```python
from build123d import *

# Parameters (mm, degrees)
SKETCH_1_W          = 200
SKETCH_1_H          = 240
SKETCH_1_R          = 3.25
EXTRUDE_1_DEPTH     = 5
FILLET_1_R          = 20
SKETCH_3_W          = 5
SKETCH_3_H          = 30
CUT_EXTRUDE_1_DEPTH = 39
SKETCH_4_R          = 1.55
CUT_EXTRUDE_2_DEPTH = 5


with BuildPart() as part:
    # 草图1 → 凸台-拉伸1 (new body)
    with BuildSketch(Plane.XY):
        Rectangle(SKETCH_1_W, SKETCH_1_H)
        with Locations((30, 30)):
            Circle(SKETCH_1_R, mode=Mode.SUBTRACT)
        with Locations(Location((30, -30, 0), (0, 0, 180))):
            Circle(SKETCH_1_R, mode=Mode.SUBTRACT)
        with Locations(Location((-30, 30, 0), (0, 0, 180))):
            Circle(SKETCH_1_R, mode=Mode.SUBTRACT)
        with Locations((-30, -30)):
            Circle(SKETCH_1_R, mode=Mode.SUBTRACT)
    extrude(amount=EXTRUDE_1_DEPTH)

    # 圆角1
    fillet_1_edges = [part.edges().sort_by_distance(p)[0] for p in [
        (-100, 120, 2.5),
        (-100, -120, 2.5),
        (100, -120, 2.5),
        (100, 120, 2.5),
    ]]
    fillet(fillet_1_edges, radius=FILLET_1_R)

    # 草图3 → 切除-拉伸1 (cut)
    with BuildSketch(Plane.XY.offset(5)):
        with Locations((97.5, 75)):
            Rectangle(SKETCH_3_W, SKETCH_3_H)
        with Locations((97.5, -30)):
            Rectangle(SKETCH_3_W, SKETCH_3_H)
        with Locations((97.5, 30)):
            Rectangle(SKETCH_3_W, SKETCH_3_H)
        with Locations((97.5, -75)):
            Rectangle(SKETCH_3_W, SKETCH_3_H)
        with Locations((-97.5, -75)):
            Rectangle(SKETCH_3_W, SKETCH_3_H)
        with Locations((-97.5, -30)):
            Rectangle(SKETCH_3_W, SKETCH_3_H)
        with Locations((-97.5, 30)):
            Rectangle(SKETCH_3_W, SKETCH_3_H)
        with Locations((-97.5, 75)):
            Rectangle(SKETCH_3_W, SKETCH_3_H)
    extrude(amount=-CUT_EXTRUDE_1_DEPTH, mode=Mode.SUBTRACT)

    # 草图4 → 切除-拉伸2 (cut)
    with BuildSketch(Plane.XY.offset(5)):
        with Locations((95, 88.45)):
            Circle(SKETCH_4_R)
        with Locations((95, 61.55)):
            Circle(SKETCH_4_R)
        with Locations((95, 43.45)):
            Circle(SKETCH_4_R)
        with Locations((95, 16.55)):
            Circle(SKETCH_4_R)
        with Locations((95, -16.55)):
            Circle(SKETCH_4_R)
        with Locations((95, -43.45)):
            Circle(SKETCH_4_R)
        with Locations((95, -61.55)):
            Circle(SKETCH_4_R)
        with Locations((95, -88.45)):
            Circle(SKETCH_4_R)
        with Locations((-95, -88.45)):
            Circle(SKETCH_4_R)
        with Locations((-95, -61.55)):
            Circle(SKETCH_4_R)
        with Locations((-95, -43.45)):
            Circle(SKETCH_4_R)
        with Locations((-95, -16.55)):
            Circle(SKETCH_4_R)
        with Locations((-95, 16.55)):
            Circle(SKETCH_4_R)
        with Locations((-95, 43.45)):
            Circle(SKETCH_4_R)
        with Locations((-95, 61.55)):
            Circle(SKETCH_4_R)
        with Locations((-95, 88.45)):
            Circle(SKETCH_4_R)
    extrude(amount=-CUT_EXTRUDE_2_DEPTH, mode=Mode.SUBTRACT)


solid = part.part
```
Geometry: final body of the model. Coordinates: model frame, mm. A direction names the side the tool comes from. Round coordinates to 2 decimals unless told otherwise and drop trailing zeros. Write each loop counter-clockwise with the first axis right and the second up, starting at its lowest first coordinate (ties: lowest second). Pieces come first, ordered by that corner, then holes. Notation, with made-up numbers: (85.5, 36) -> (142.5, 36) arc R8 cw to (142.5, 42) -> close; hole circle Ø3 at (81, 48.25). An arc over 180 degrees is marked (long way). Use CSV: the item, a comma, the result in double quotes. Start each with the question number.
Q1. Line query: L1, parallel to Y at x = -30, z = 2.6; L2, parallel to Y at x = -28, z = 2.65; L3, parallel to X at y = -69.5, z = 3.5. Output: solid intervals per line, ascending.
Q2. Section B-B (x = 30). Return loops of the section in (y, z).
Q3. Section A-A (y = -30). Return loops of the section in (x, z).
Q4. Section D-D (y = 36). Return loops of the section in (x, z), plus the area to 3 significant figures.
Q5. Reachability of faces 5 (the face through (-100, 95, 2)), 6 (the face through (-98, -60, 3)), 7 (the face through (97, 60, 3)) from +Z, -Z, +X, -X, +Y, -Y: full face, straight path, thin tool, end or side. Return the list, or none.
Q6. Pull-direction query (Y, two-part tool) for faces 1 (the face through (93.986, -114.297, 2.535)), 2 (the face through (100, 0, 2)), 3 (the face through (28.5, -27.117, 2.465)), 4 (the face through (-95, 30, 3)); classes: pulls with the +Y half, pulls with the -Y half, needs draft (parallel to the pull), parting line crosses it, or undercut.
Q7. Section C-C (z = 4). Give the number of separate pieces and of enclosed holes in the cut face, plus the area to 3 significant figures.
Q8. First-contact query: pin 1 Ø4 at (x, y) = (-30, 30) entering from +Z; pin 2 Ø1.5 at (x, z) = (97, 3) entering from -Y; pin 3 Ø2.5 at (x, z) = (98, 2.5) entering from -Y; pin 4 Ø1.5 at (x, z) = (98, 2.5) entering from +Y. Flat tips, straight axial feed; report the tip coordinate or a pass-through.
Result sheet:
1,L1,"-120 to -33.25, -26.75 to 26.75, 33.25 to 120"
1,L2,"-120 to -32.56, -27.44 to 27.44, 32.56 to 120"
1,L3,"-95 to 95"
2,outline,"(-120, 0) -> (-33.25, 0) -> (-33.25, 5) -> (-120, 5) -> close; (-26.75, 0) -> (26.75, 0) -> (26.75, 5) -> (-26.75, 5) -> close; (33.25, 0) -> (120, 0) -> (120, 5) -> (33.25, 5) -> close"
3,outline,"(-95, 0) -> (-33.25, 0) -> (-33.25, 5) -> (-95, 5) -> close; (-26.75, 0) -> (26.75, 0) -> (26.75, 5) -> (-26.75, 5) -> close; (33.25, 0) -> (95, 0) -> (95, 5) -> (33.25, 5) -> close"
4,outline,"(-95, 0) -> (95, 0) -> (95, 5) -> (-95, 5) -> close"
4,area,"950 mm²"
5,face 5,"+Z, -Z, -X, +Y, -Y"
5,face 6,"+Z, -Z, -X"
5,face 7,"+Z, -Z, +X"
6,face 1,"pulls with the -Y half"
6,face 2,"needs draft"
6,face 3,"undercut"
6,face 4,"undercut"
7,separate pieces,"1"
7,enclosed holes,"4"
7,area,"46,300 mm²"
8,pin 1,"through"
8,pin 2,"y = -111.66"
8,pin 3,"y = -110.93"
8,pin 4,"y = 110.12"
